Verification items for this drawing (mm, ordinates from the low corner). A direction names the side the tool comes from. Give positions to 0.01 mm unless a question says otherwise; leave off trailing zeros. Write each loop counter-clockwise with the first axis right and the second up, starting at its lowest first coordinate (ties: lowest second). Pieces come first, ordered by that corner, then holes. Notation, with made-up numbers: M 29.25,77.5 L 48.25,77.5 A25 cw 48.25,101.5 Z; hole C 15,-20.75 d1. An arc over 180 degrees is marked long. Use one line per item in the form item = value. Start each with the question number.
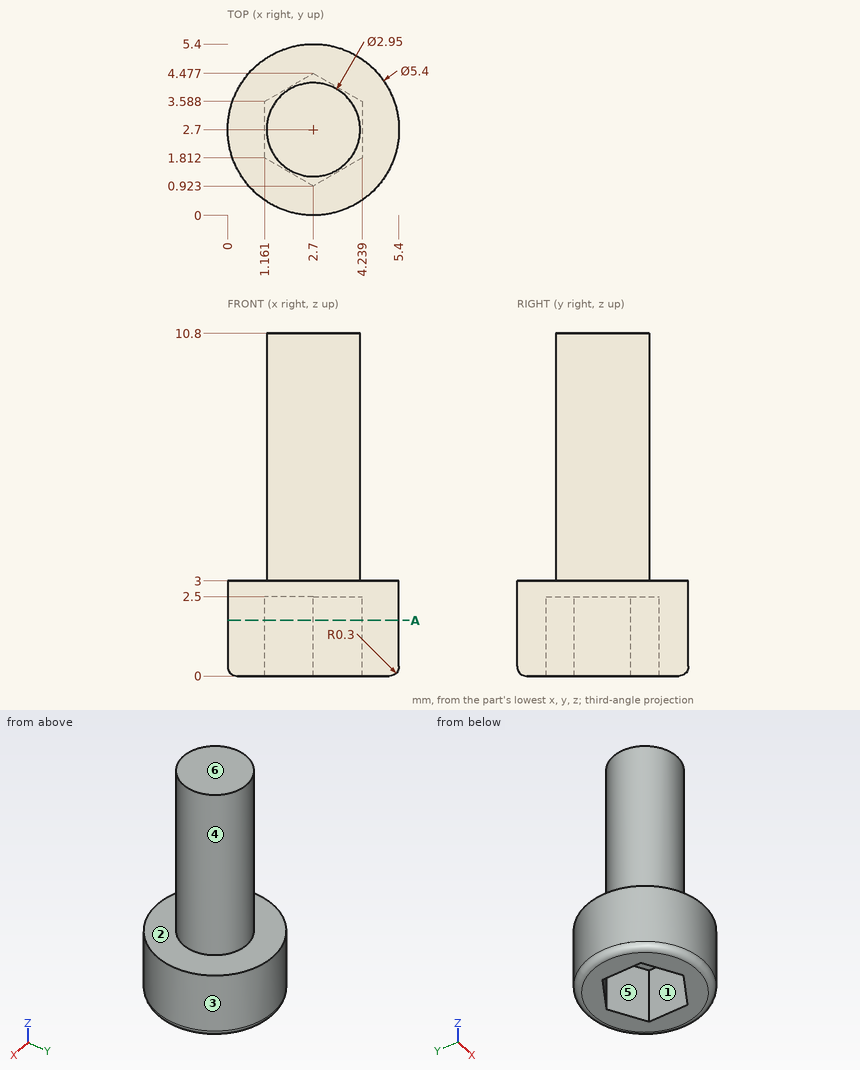
(1) Draft check along Y on the marked faces 1, 2 and 3. Enter one of: released by +Y, released by -Y, zero draft, split by the parting line, or undercut.
(2) Tool access check on the marked faces 4, 5 and 6. Record the directions out of +Z, -Z, +X, -X, +Y, -Y that give a thin tool (end or side, any length) a straight path to the whole face; none if there is none.
(3) Sectioned sample at A-A, the plane z = 1.75. Record the boundary of the cut face in (x, y), plus the area to 3 significant figures.
(4) Depth check by flat-ended pin: pin 1 (1.5 mm diameter, centred on x = 2.5, y = 3, fed in from -Z). Enter the tip coordinate at first touch or a pass-through.
(5) Thickness scan on probe 1 along Z at (x, y) = (2.2, 4.45); probe 2 along Y at (x, z) = (2.7, 9.25) (1 decimal); probe 3 along Z at (x, y) = (2.6, 3.7). Record the ranges inside material, lowest first. Write a range as [from, to].
Numbers:
q1.face_1 = undercut
q1.face_2 = zero draft
q1.face_3 = split by the parting line
q2.face_4 = +Z
q2.face_5 = -Z
q2.face_6 = +Z, +X, -X, +Y, -Y
q3.outline = C 2.7,2.7 d5.4; hole M 1.16,1.81 L 2.7,0.92 L 4.24,1.81 L 4.24,3.59 L 2.7,4.48 L 1.16,3.59 Z
q3.area = 14.7 mm2
q4.pin_1 = 2.5
q5.probe_1 = [0, 3]
q5.probe_2 = [1.2, 4.2]
q5.probe_3 = [2.5, 10.8]
